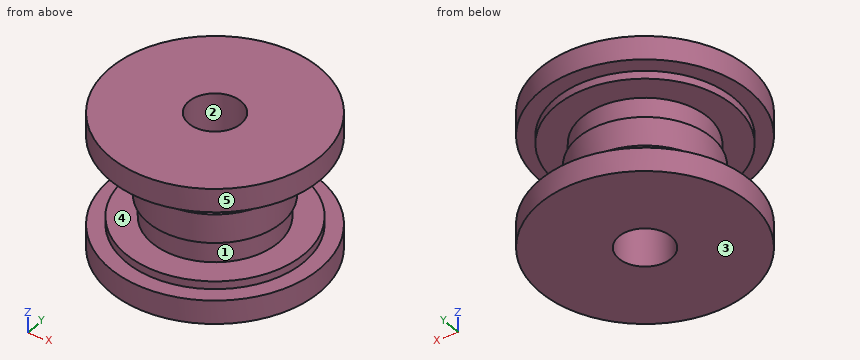
from build123d import *

# Parameters (mm, degrees)
F0_R      = 20
F1_DEPTH  = 4.5
F2_R      = 17
F3_DEPTH  = 1.5
F4_R      = 12
F5_DEPTH  = 4.25
F6_R      = 12.75
F7_DEPTH  = 5.5
F8_R      = 12
F9_DEPTH  = 4.25
F10_R     = 17
F11_DEPTH = 1.5
F12_R     = 20
F13_DEPTH = 4.5
F14_R     = 5
F15_DEPTH = 30


with BuildPart() as f1:
    # F0 (on Top) → F1 (new body)
    with BuildSketch(Plane.XY):
        Circle(F0_R)
    extrude(amount=F1_DEPTH)

    # F2 (on face) → F3 (join)
    with BuildSketch(Plane.XY.offset(4.5)):
        Circle(F2_R)
    extrude(amount=F3_DEPTH)

    # F4 (on face) → F5 (join)
    with BuildSketch(Plane.XY.offset(6)):
        Circle(F4_R)
    extrude(amount=F5_DEPTH)

    # F6 (on face) → F7 (join)
    with BuildSketch(Plane.XY.offset(10.25)):
        Circle(F6_R)
    extrude(amount=F7_DEPTH)

    # F8 (on face) → F9 (join)
    with BuildSketch(Plane.XY.offset(15.75)):
        Circle(F8_R)
    extrude(amount=F9_DEPTH)

    # F10 (on face) → F11 (join)
    with BuildSketch(Plane.XY.offset(20)):
        Circle(F10_R)
    extrude(amount=F11_DEPTH)

    # F12 (on face) → F13 (join)
    with BuildSketch(Plane.XY.offset(21.5)):
        Circle(F12_R)
    extrude(amount=F13_DEPTH)

    # F14 (on face) → F15 (cut)
    with BuildSketch(Plane.XY.offset(26)):
        Circle(F14_R)
    extrude(amount=-F15_DEPTH, mode=Mode.SUBTRACT)


solid = f1.part
CAD build for the part. Positions are in the model's coordinates, mm. Face numbers are marked on the shaded views. A direction names the side the tool comes from. Coordinates: 2 decimals unless noted, no trailing zeros. Write each loop counter-clockwise with the first axis right and the second up, starting at its lowest first coordinate (ties: lowest second). Pieces come first, ordered by that corner, then holes. Notation, with made-up numbers: M 18.5,19 L 62.5,19 A14 cw 62.5,24 Z; hole C -22.5,2.5 d11. An arc over 180 degrees is marked long. Answer as a JSON object with one key per item and string values. Group by question number.
1) Saw through at D-D (y = -6). Write the cut outline in (x, z).
2) Pin check, flat tips, straight feed: pin 1 Ø3 at (y, z) = (-13.5, 20.5) entering from -X; pin 2 Ø3 at (x, z) = (-11, 18) entering from -Y; pin 3 Ø3 at (x, z) = (11, 15.5) entering from -Y; pin 4 Ø8 at (x, y) = (0, 0) entering from +Z. Stop position of each tip, or through.
3) Wall check: line 1 (Z direction, x = -9, y = 15); line 2 (Y direction, x = 0, z = 10.5); line 3 (Y direction, x = 0, z = 18.5). Give the ranges that are in metal, low to high. Write a range as from..to.
4) Saw through at C-C (z = 14.25). Write the cut outline in (x, y).
5) Mould opens along X. For the marked faces 1, 2 and 3 say: +X half, -X half, draft (parallel to the pull), parting line (faces both ways), or undercut.
6) Tool access for the marked faces 4 and 5: list every direction of +Z, -Z, +X, -X, +Y, -Y with a clear straight run to the whole face (end or side of a thin tool).
Values follow:
{
 "1": {"outline": "M -19.08,0 L 19.08,0 L 19.08,4.5 L 15.91,4.5 L 15.91,6 L 10.39,6 L 10.39,10.25 L 11.25,10.25 L 11.25,15.75 L 10.39,15.75 L 10.39,20 L 15.91,20 L 15.91,21.5 L 19.08,21.5 L 19.08,26 L -19.08,26 L -19.08,21.5 L -15.91,21.5 L -15.91,20 L -10.39,20 L -10.39,15.75 L -11.25,15.75 L -11.25,10.25 L -10.39,10.25 L -10.39,6 L -15.91,6 L -15.91,4.5 L -19.08,4.5 Z"},
 "2": {"pin 1": "stops at x = -15.71", "pin 2": "stops at y = -7.33", "pin 3": "stops at y = -8.5", "pin 4": "passes through"},
 "3": {"line 1": "z = 0..4.5, 21.5..26", "line 2": "y = -12.75..-5, 5..12.75", "line 3": "y = -12..-5, 5..12"},
 "4": {"outline": "C 0,0 d25.5; hole C 0,0 d10"},
 "5": {"face 1": "parting line", "face 2": "undercut", "face 3": "draft"},
 "6": {"face 4": "none", "face 5": "+Z, -Z"}
}
